```python
from build123d import *

# Parameters (mm, degrees)
ESQUISSE1_W        = 25
ESQUISSE1_H        = 14.5
BOSS_EXTRU_1_DEPTH = 1
ESQUISSE2_W        = 3.8
ESQUISSE2_H        = 5
BOSS_EXTRU_2_DEPTH = 2
ESQUISSE2_3_W      = 5
ESQUISSE2_3_H      = 5
BOSS_EXTRU_3_DEPTH = 1
BOSS_EXTRU_4_START = -1
ESQUISSE2_4_W      = 5
ESQUISSE2_4_H      = 10
BOSS_EXTRU_4_DEPTH = 2.5
BOSS_EXTRU_5_START = -3.5
ESQUISSE2_5_W      = 0.8
ESQUISSE2_5_H      = 0.8
BOSS_EXTRU_5_DEPTH = 6.5
ESQUISSE2_6_W      = 0.8
ESQUISSE2_6_H      = 0.8
BOSS_EXTRU_6_DEPTH = 2


with BuildPart() as part:
    # Esquisse1 → Boss.-Extru.1 (new body)
    with BuildSketch(Plane(origin=(0, 0, 0), x_dir=(1, 0, 0), z_dir=(0, 1, 0))):
        with Locations((-12.5, -7.25)):
            Rectangle(ESQUISSE1_W, ESQUISSE1_H)
    extrude(amount=BOSS_EXTRU_1_DEPTH)

    # Esquisse2 → Boss.-Extru.2 (add)
    with BuildSketch(Plane(origin=(0, 1, 0), x_dir=(1, 0, 0), z_dir=(0, 1, 0))):
        with Locations((-15.1, -11.8)):
            Rectangle(ESQUISSE2_W, ESQUISSE2_H)
    extrude(amount=BOSS_EXTRU_2_DEPTH)

    # Esquisse2<3> → Boss.-Extru.3 (add)
    with BuildSketch(Plane(origin=(0, 1, 0), x_dir=(1, 0, 0), z_dir=(0, 1, 0))):
        with Locations((-15.5, -5.5)):
            Rectangle(ESQUISSE2_3_W, ESQUISSE2_3_H)
    extrude(amount=BOSS_EXTRU_3_DEPTH)

    # Esquisse2<4> → Boss.-Extru.4 (add)
    with BuildSketch(Plane(origin=(0, 1, 0), x_dir=(1, 0, 0), z_dir=(0, 1, 0)).offset(BOSS_EXTRU_4_START)):
        with Locations((-22.5, -7.25)):
            Rectangle(ESQUISSE2_4_W, ESQUISSE2_4_H)
    extrude(amount=-BOSS_EXTRU_4_DEPTH)

    # Esquisse2<5> → Boss.-Extru.5 (add)
    with BuildSketch(Plane(origin=(0, 1, 0), x_dir=(1, 0, 0), z_dir=(0, 1, 0)).offset(BOSS_EXTRU_5_START)):
        with Locations((-23.8, -3.45)):
            Rectangle(ESQUISSE2_5_W, ESQUISSE2_5_H)
        with Locations((-21.2, -3.45)):
            Rectangle(ESQUISSE2_5_W, ESQUISSE2_5_H)
        with Locations((-21.2, -6.05)):
            Rectangle(ESQUISSE2_5_W, ESQUISSE2_5_H)
        with Locations((-21.2, -8.65)):
            Rectangle(ESQUISSE2_5_W, ESQUISSE2_5_H)
        with Locations((-21.2, -11.25)):
            Rectangle(ESQUISSE2_5_W, ESQUISSE2_5_H)
        with Locations((-23.8, -11.25)):
            Rectangle(ESQUISSE2_5_W, ESQUISSE2_5_H)
        with Locations((-23.8, -6.05)):
            Rectangle(ESQUISSE2_5_W, ESQUISSE2_5_H)
        with Locations((-23.8, -8.65)):
            Rectangle(ESQUISSE2_5_W, ESQUISSE2_5_H)
    extrude(amount=-BOSS_EXTRU_5_DEPTH)

    # Esquisse2<6> → Boss.-Extru.6 (add)
    with BuildSketch(Plane(origin=(0, 1, 0), x_dir=(1, 0, 0), z_dir=(0, 1, 0))):
        with Locations((-23.8, -3.45)):
            Rectangle(ESQUISSE2_6_W, ESQUISSE2_6_H)
        with Locations((-21.2, -3.45)):
            Rectangle(ESQUISSE2_6_W, ESQUISSE2_6_H)
        with Locations((-21.2, -6.05)):
            Rectangle(ESQUISSE2_6_W, ESQUISSE2_6_H)
        with Locations((-23.8, -6.05)):
            Rectangle(ESQUISSE2_6_W, ESQUISSE2_6_H)
        with Locations((-23.8, -8.65)):
            Rectangle(ESQUISSE2_6_W, ESQUISSE2_6_H)
        with Locations((-21.2, -8.65)):
            Rectangle(ESQUISSE2_6_W, ESQUISSE2_6_H)
        with Locations((-21.2, -11.25)):
            Rectangle(ESQUISSE2_6_W, ESQUISSE2_6_H)
        with Locations((-23.8, -11.25)):
            Rectangle(ESQUISSE2_6_W, ESQUISSE2_6_H)
    extrude(amount=BOSS_EXTRU_6_DEPTH)


solid = part.part
```
The model under review builds one solid part; all positions refer to its coordinate system, in mm. A direction names the side the tool comes from. Round coordinates to 2 decimals unless told otherwise and drop trailing zeros. Loops run counter-clockwise (first coordinate to the right, second up) from the corner with the lowest first, then second, coordinate; pieces in that order, holes last. Notation, with made-up numbers: (-1, -32.75) - (36, -32.75) arc R11 ccw to (36, -24.75) - close; hole circle Ø8 at (-28, -16). An arc over 180 degrees is marked (long way). Use a Markdown table: item, result. Add a question column.
Q1. Insertion check: pin 1 Ø0.9 at (y, z) = (-6, 6) entering from +X; pin 2 Ø3 at (x, z) = (-21.5, 2.5) entering from -Y; pin 3 Ø0.6 at (y, z) = (2, 8.5) entering from -X; pin 4 Ø0.6 at (x, y) = (-21, 2) entering from +Z. Each pin has a flat end and moves straight along its axis. Give the tip position at first contact, or say it passes through.
Q2. For probe 1 along Z at (x, y) = (-21.5, -2.75); probe 2 along X at (y, z) = (-5.5, 11.25); probe 3 along Y at (x, z) = (-13.25, 1.25), list the stretches that pass through material, from the lowest coordinate up.
Q3. The part is to be moulded in two halves that separate along X. For faces 6 (the face through (-24.2, 2, 8.7)), 7 (the face through (-20.8, 2, 8.7)), 8 (the face through (-23.4, -6, 11)), 9 (the face through (-12.7, 0.5, 14.5)), say which applies: pulls with the +X half, pulls with the -X half, needs draft (parallel to the pull), parting line crosses it, or undercut.
Q4. Machinability: for faces 1 (the face through (-15.5, 1.5, 3)), 2 (the face through (-24.2, 2, 11)), 3 (the face through (-18, 1.5, 5.5)), 4 (the face through (-23.4, -5.7, 8.7)), 5 (the face through (-24.2, -5.7, 8.7)), which of the approach directions +Z, -Z, +X, -X, +Y, -Y give a long, thin tool a straight path to every point of the face, cutting with its end or side? Answer none if there is none.
Q5. Add section B-B (x = -15.75). State the section outline as (y, z) points.
Q6. Add section A-A (y = -6). State how many separate pieces and enclosed holes the cut face has, plus the area to 3 significant figures.
Q7. Add section C-C (z = 12.75). State the section outline as (x, y) points, plus the area to 3 significant figures.
Q8. Add section D-D (y = -0.5). State the section outline as (x, z) points, plus the area to 3 significant figures.
Worked answers:
| question | item | result |
|---|---|---|
| 1 | pin 1 | x = -20.8 |
| 1 | pin 2 | y = -9 |
| 1 | pin 3 | x = -24.2 |
| 1 | pin 4 | z = 11.65 |
| 2 | probe 1 | 3.05 to 3.85, 5.65 to 6.45, 8.25 to 9.05, 10.85 to 11.65 |
| 2 | probe 2 | -24.2 to -23.4, -21.6 to -20.8 |
| 2 | probe 3 | 0 to 1 |
| 3 | face 6 | pulls with the -X half |
| 3 | face 7 | pulls with the +X half |
| 3 | face 8 | undercut |
| 3 | face 9 | needs draft |
| 4 | face 1 | -Z, +X, -X, +Y |
| 4 | face 2 | +Z, -Z, -X, +Y |
| 4 | face 3 | +Z, -Z, +Y |
| 4 | face 4 | +Z, -Z, -Y |
| 4 | face 5 | +Z, -Z, -X, -Y |
| 5 | outline | (0, 0) - (1, 0) - (1, 3) - (2, 3) - (2, 8) - (1, 8) - (1, 9.3) - (3, 9.3) - (3, 14.3) - (1, 14.3) - (1, 14.5) - (0, 14.5) - close |
| 6 | separate pieces | 8 |
| 6 | enclosed holes | 0 |
| 6 | area | 5.12 mm² |
| 7 | outline | (-25, 0) - (0, 0) - (0, 1) - (-13.2, 1) - (-13.2, 3) - (-17, 3) - (-17, 1) - (-25, 1) - close |
| 7 | area | 32.6 mm² |
| 8 | outline | (-25, 2.25) - (-20, 2.25) - (-20, 12.25) - (-25, 12.25) - close |
| 8 | area | 50.0 mm² |
